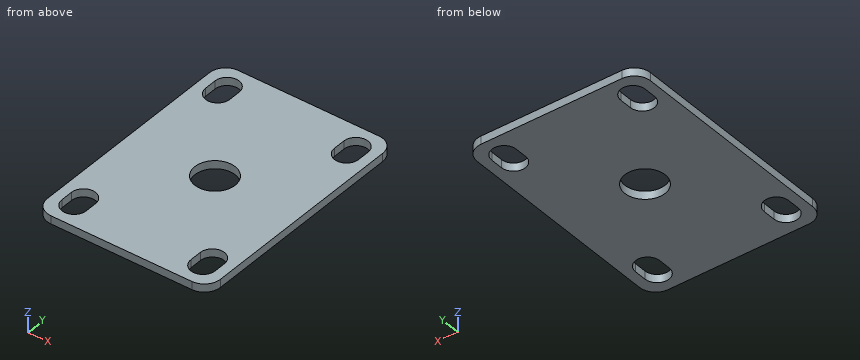
```python
from build123d import *

# Parameters (mm, degrees)
SKETCH1_R           = 5
BOSS_EXTRUDE1_DEPTH = 2


with BuildPart() as part:
    # Sketch1 → Boss-Extrude1 (new body)
    with BuildSketch(Plane.XY):
        with BuildLine():
            Line((4, 0), (39, 0))
            ThreePointArc((39, 0), (41.828427125, 1.171572875), (43, 4))
            Line((43, 4), (43, 56))
            ThreePointArc((43, 56), (41.828427125, 58.828427125), (39, 60))
            Line((39, 60), (4, 60))
            ThreePointArc((4, 60), (1.171572875, 58.828427125), (0, 56))
            Line((0, 56), (0, 4))
            ThreePointArc((0, 4), (1.171572875, 1.171572875), (4, 0))
        make_face()
        with Locations((21.5, 30)):
            Circle(SKETCH1_R, mode=Mode.SUBTRACT)
        with BuildLine():
            Line((40.5, 8.5), (40.5, 5.5))
            ThreePointArc((40.5, 5.5), (37.5, 2.5), (34.5, 5.5))
            Line((34.5, 5.5), (34.5, 8.5))
            ThreePointArc((34.5, 8.5), (37.5, 11.5), (40.5, 8.5))
        make_face(mode=Mode.SUBTRACT)
        with BuildLine():
            Line((40.5, 51.5), (40.5, 54.5))
            ThreePointArc((40.5, 54.5), (37.5, 57.5), (34.5, 54.5))
            Line((34.5, 54.5), (34.5, 51.5))
            ThreePointArc((34.5, 51.5), (37.5, 48.5), (40.5, 51.5))
        make_face(mode=Mode.SUBTRACT)
        with BuildLine():
            Line((2.5, 8.5), (2.5, 5.5))
            ThreePointArc((2.5, 5.5), (5.5, 2.5), (8.5, 5.5))
            Line((8.5, 5.5), (8.5, 8.5))
            ThreePointArc((8.5, 8.5), (5.5, 11.5), (2.5, 8.5))
        make_face(mode=Mode.SUBTRACT)
        with BuildLine():
            Line((2.5, 51.5), (2.5, 54.5))
            ThreePointArc((2.5, 54.5), (5.5, 57.5), (8.5, 54.5))
            Line((8.5, 54.5), (8.5, 51.5))
            ThreePointArc((8.5, 51.5), (5.5, 48.5), (2.5, 51.5))
        make_face(mode=Mode.SUBTRACT)
    extrude(amount=BOSS_EXTRUDE1_DEPTH)


solid = part.part
```
Input: part model. Units: mm. Frame: model coordinates. Give positions to 0.01 mm unless a question says otherwise; leave off trailing zeros. Write each loop counter-clockwise with the first axis right and the second up, starting at its lowest first coordinate (ties: lowest second). Pieces come first, ordered by that corner, then holes. Notation, with made-up numbers: (-17, 0) - (39, 0) arc R20 ccw to (39, 17) - close; hole circle Ø11 at (-2.5, 53). An arc over 180 degrees is marked (long way). Write item = value, one per line. Start each with the question number.
1. Section query C-C, the plane x = 37.5. Output: boundary loops of the cut face in (y, z), then the cut area to 3 significant figures.
2. Section query B-B, the plane x = 21.5. Output: boundary loops of the cut face in (y, z), then the cut area to 3 significant figures.
3. Ray query, L1, parallel to Y at x = 37.5, z = 1.4; L2, parallel to X at y = 53.5, z = 1.35; L3, parallel to Y at x = 21.5, z = 0.8. Return the intervals inside material, ascending.
4. Section query D-D, the plane z = 1.7. Output: boundary loops of the cut face in (x, y), then the cut area to 3 significant figures.
5. First-contact query: pin 1 Ø13 at (x, y) = (21.5, 30) entering from +Z. Flat tip, straight axial feed; report the tip coordinate or a pass-through.
6. Section query A-A, the plane y = 30. Output: boundary loops of the cut face in (x, z).
Check sheet entries:
q1.outline = (0, 0) - (2.5, 0) - (2.5, 2) - (0, 2) - close; (11.5, 0) - (48.5, 0) - (48.5, 2) - (11.5, 2) - close; (57.5, 0) - (60, 0) - (60, 2) - (57.5, 2) - close
q1.area = 84.0 mm2
q2.outline = (0, 0) - (25, 0) - (25, 2) - (0, 2) - close; (35, 0) - (60, 0) - (60, 2) - (35, 2) - close
q2.area = 100 mm2
q3.L1 = 0 to 2.5, 11.5 to 48.5, 57.5 to 60
q3.L2 = 0 to 2.5, 8.5 to 34.5, 40.5 to 43
q3.L3 = 0 to 25, 35 to 60
q4.outline = (0, 4) arc R4 ccw to (4, 0) - (39, 0) arc R4 ccw to (43, 4) - (43, 56) arc R4 ccw to (39, 60) - (4, 60) arc R4 ccw to (0, 56) - close; hole (2.5, 5.5) arc R3 ccw to (8.5, 5.5) - (8.5, 8.5) arc R3 ccw to (2.5, 8.5) - close; hole (2.5, 51.5) arc R3 ccw to (8.5, 51.5) - (8.5, 54.5) arc R3 ccw to (2.5, 54.5) - close; hole circle Ø10 at (21.5, 30); hole (34.5, 5.5) arc R3 ccw to (40.5, 5.5) - (40.5, 8.5) arc R3 ccw to (34.5, 8.5) - close; hole (34.5, 51.5) arc R3 ccw to (40.5, 51.5) - (40.5, 54.5) arc R3 ccw to (34.5, 54.5) - close
q4.area = 2,300 mm2
q5.pin_1 = 2
q6.outline = (0, 0) - (16.5, 0) - (16.5, 2) - (0, 2) - close; (26.5, 0) - (43, 0) - (43, 2) - (26.5, 2) - close
